Study the drawing (mm; zero at the part's minimum x, y, z) and answer. Give positions to 0.01 mm unless a question says otherwise; leave off trailing zeros. Loops run counter-clockwise (first coordinate to the right, second up) from the corner with the lowest first, then second, coordinate; pieces in that order, holes last. Notation, with made-up numbers: (21, 49) - (59, 49) arc R18 cw to (59, 66) - close; hole circle Ø4 at (39.5, 89). An arc over 180 degrees is marked (long way). Write item = value, one per line. Start each with the question number.
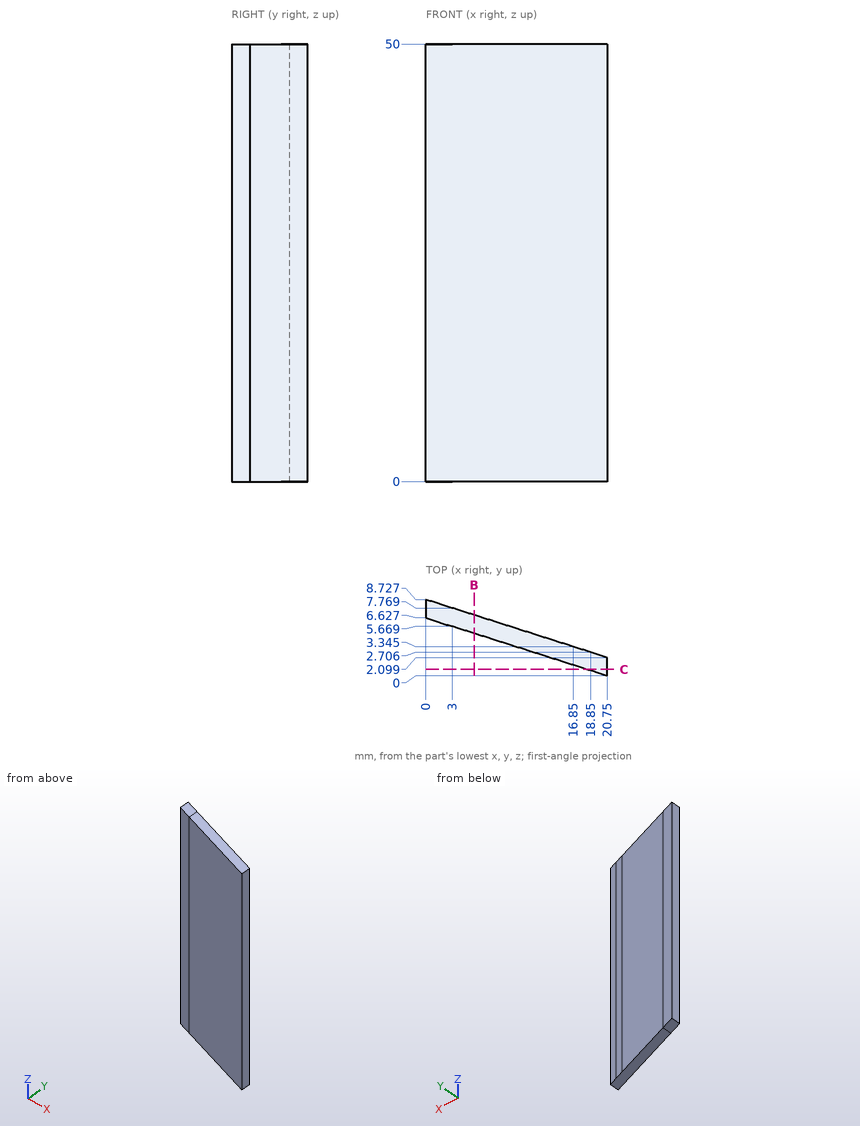
1. A cutting plane is placed at C-C on y = 0.75. Give the vertices of the cut face in (x, z).
2. A cutting plane is placed at B-B on x = 5.5. Give the vertices of the cut face in (y, z), and give its area (3 significant figures).
3. Consider line 1 along Y through (x, z) = (8.75, 32.5); line 2 along Y through (x, z) = (8, 28). Determine where each line is inside the solid, lowest interval first. Write a range as [from, to].
Reply:
q1.outline = (18.4, 0) - (20.75, 0) - (20.75, 50) - (18.4, 50) - close
q2.outline = (4.87, 0) - (6.97, 0) - (6.97, 50) - (4.87, 50) - close
q2.area = 105 mm^2
q3.line_1 = [3.83, 5.93]
q3.line_2 = [4.07, 6.17]
